```python
from build123d import *

# Parameters (mm, degrees)
CUT_EXTRUDE1_DEPTH = 15


with BuildPart() as part:
    # Sketch1 → Revolve1 (revolve)
    with BuildSketch(Plane.XY, mode=Mode.PRIVATE) as revolve1_sk:
        Polygon((0, 0), (27, 0), (27, 2.5), (12, 2.5), (12, 3.1), (3, 3.1), (3, 5), (0, 5), align=None)
    revolve(revolve1_sk.sketch.rotate(Axis((0, 0, 0), (1, 0, 0)), 90), axis=Axis((0, 0, 0), (1, 0, 0)))

    # Sketch2 → Cut-Extrude1 (cut)
    with BuildSketch(Plane(origin=(27, 0, 0), x_dir=(0, 0, -1), z_dir=(1, 0, 0))):
        Polygon((-1.1, 2.244994432), (-1.1, 0.544994432), (1.1, 0.544994432), (1.1, 2.244994432), (0, 3.059798295), align=None)
    extrude(amount=-CUT_EXTRUDE1_DEPTH, mode=Mode.SUBTRACT)


solid = part.part
```
Here's how the part is built. I have some questions about the finished solid (model axes, mm). A direction names the side the tool comes from. Give positions to 0.01 mm unless a question says otherwise; leave off trailing zeros. Write each loop counter-clockwise with the first axis right and the second up, starting at its lowest first coordinate (ties: lowest second). Pieces come first, ordered by that corner, then holes.
(1) On a 3-axis mill with a long thin cutter (end or side, diameter ignored), from which of +Z, -Z, +X, -X, +Y, -Y can I reach the whole of each face in a straight line? I mean faces 4 (the face through (20, 1, 1.1)), 5 (the face through (7.437, -0.931, 2.957)), 6 (the face through (1, 0, -5)). Say none if no direction works.
Output values:
face 4: +X, +Y
face 5: +X
face 6: +X, -X
(2) Imagine slicing it at B-B, the plane y = 0. Write out the boundary of the cut face in (x, z).
Output values:
outline: (0, -5) - (3, -5) - (3, -3.1) - (12, -3.1) - (12, -2.5) - (27, -2.5) - (27, 2.5) - (12, 2.5) - (12, 3.1) - (3, 3.1) - (3, 5) - (0, 5) - close
(3) If I drill on L1, parallel to X at y = -3.25, z = -2.75; L2, parallel to X at y = -1.75, z = 2.5; L3, parallel to Z at x = 6, y = 0.25, over which ranges is the centre line in solid material (lowest first)?
Output values:
L1: x = 0 to 3
L2: x = 0 to 12
L3: z = -3.09 to 3.09
(4) Thinking about a two-plate mould opening in Z: for faces 1 (the face through (19.4, -2.5, 0.1)), 2 (the face through (0, 0, 0)), 3 (the face through (20, 1, -1.1)), which applies, pulls with the +Z half, pulls with the -Z half, needs draft (parallel to the pull), parting line crosses it, or undercut?
Output values:
face 1: parting line crosses it
face 2: needs draft
face 3: undercut
(5) Imagine slicing it at D-D, the plane y = 2.5. Write out the boundary of the cut face in (x, z).
Output values:
outline: (0, -4.33) - (3, -4.33) - (3, -1.83) - (12, -1.83) - (12, 1.83) - (3, 1.83) - (3, 4.33) - (0, 4.33) - close
(6) Imagine slicing it at A-A, the plane z = 0. Write out the boundary of the cut face in (x, y) (3 decimals), and give its area (3 significant figures).
Output values:
outline: (0, -5) - (3, -5) - (3, -3.1) - (12, -3.1) - (12, -2.5) - (27, -2.5) - (27, 0.545) - (12, 0.545) - (12, 3.1) - (3, 3.1) - (3, 5) - (0, 5) - close
area: 131 mm2
(7) Will these pins go through, and if not, where does the flat tip stop? pin 1 (1.9 mm diameter, centred on x = 22, y = 1.5, fed in from +Z); pin 2 (5 mm diameter, centred on x = 4.5, z = 3, fed in from -Y); pin 3 (1 mm diameter, centred on x = 16, z = -0.5, fed in from -Y); pin 4 (6 mm diameter, centred on y = -3.5, z = 2.5, fed in from +X).
Output values:
pin 1: stops at z = 2.44
pin 2: stops at y = -4.9
pin 3: stops at y = -2.5
pin 4: stops at x = 27
(8) Imagine slicing it at C-C, the plane x = 19.75. Write out the boundary of the cut face in (y, z) (3 decimals), and give its area (3 significant figures).
Output values:
outline: (0.545, -1.1) - (0.545, 1.1) - (2.245, 1.1) arc R2.5 ccw (long way) to (2.245, -1.1) - close
area: 15.5 mm2
